Could you check a few things on this model? Use its own coordinates, in mm. Face numbers are marked on the shaded views. A direction names the side the tool comes from. Coordinates: 2 decimals unless noted, no trailing zeros. Loops run counter-clockwise (first coordinate to the right, second up) from the corner with the lowest first, then second, coordinate; pieces in that order, holes last. Notation, with made-up numbers: (56, -16.5) - (79, -16.5) arc R22 cw to (79, -1.5) - close; hole circle Ø2 at (48.25, -29). An arc over 180 degrees is marked (long way). Put each result on its own line as item: value. Start each with the question number.
```python
from build123d import *

# Parameters (mm, degrees)
EXTRUDE_1_DEPTH     = 1.5
EXTRUDE_2_DEPTH     = 3
SKETCH_5_R          = 1.25
CUT_EXTRUDE_2_DEPTH = 2.5000001
CUT_EXTRUDE_3_DEPTH = 2.5000001


with BuildPart() as part:
    # Эскиз1 → Бобышка-Вытянуть1 (new body)
    with BuildSketch(Plane(origin=(0, 0, 0), x_dir=(1, 0, 0), z_dir=(0, 1, 0))):
        with BuildLine():
            Line((5, 14.5), (-5, 14.5))
            ThreePointArc((-5, 14.5), (-9.453000697, 12.420644275), (-13, 9.018919508))
            Line((-13, 9.018919508), (-13, 6.5))
            add(Edge.make_bspline(
                [(-13, 6.5), (-7.441418368, 0), (-13, -6.5)],
                knots=[0, 0, 0, 1, 1, 1], degree=2))
            Line((-13, -6.5), (-13, -9.018919508))
            ThreePointArc((-13, -9.018919508), (-9.453000697, -12.420644275), (-5, -14.5))
            Line((-5, -14.5), (5, -14.5))
            ThreePointArc((5, -14.5), (15.997963501, 0), (5, 14.5))
        make_face()
    extrude(amount=EXTRUDE_1_DEPTH)

    # Эскиз3 → Бобышка-Вытянуть2 (add)
    with BuildSketch(Plane(origin=(0, 1.5, 0), x_dir=(1, 0, 0), z_dir=(0, 1, 0))):
        with BuildLine():
            Line((4.668952027, -11), (7.497379152, -8.171572875))
            Line((7.497379152, -8.171572875), (7.497379152, 8.171572875))
            Line((7.497379152, 8.171572875), (4.668952027, 11))
            Line((4.668952027, 11), (-5.566129175, 11))
            Line((-5.566129175, 11), (-7.502620848, 7.5))
            add(Edge.make_bspline(
                [(-7.502620848, 7.5), (-4.502620848, 0), (-7.502620848, -7.5)],
                knots=[0, 0, 0, 1, 1, 1], degree=2))
            Line((-7.502620848, -7.5), (-5.566129175, -11))
            Line((-5.566129175, -11), (4.668952027, -11))
        make_face()
    extrude(amount=EXTRUDE_2_DEPTH)

    # Эскиз5 → Вырез-Вытянуть2 (cut, through all)
    with BuildSketch(Plane(origin=(0, 1.5, 0), x_dir=(1, 0, 0), z_dir=(0, 1, 0))):
        with Locations((9.863113254, 10.081034519)):
            Circle(SKETCH_5_R)
        with Locations((-10.997789514, 8.218757238)):
            Circle(SKETCH_5_R)
        with Locations((9.863113254, -10.081034519)):
            Circle(SKETCH_5_R)
        with Locations((-10.997789514, -8.218757238)):
            Circle(SKETCH_5_R)
    extrude(amount=-CUT_EXTRUDE_2_DEPTH, mode=Mode.SUBTRACT)

    # Эскиз7 → Вырез-Вытянуть3 (cut, through all)
    with BuildSketch(Plane(origin=(0, 1.5, 0), x_dir=(1, 0, 0), z_dir=(0, 1, 0))):
        with BuildLine():
            Line((-13, 9.018919508), (-13, 6.5))
            Line((-13, 6.5), (-12.715649732, 6.077566297))
            ThreePointArc((-12.715649732, 6.077566297), (-8.737112762, 11.411761045), (-2.842609373, 14.5))
            Line((-2.842609373, 14.5), (-5, 14.5))
            ThreePointArc((-5, 14.5), (-9.453000697, 12.420644275), (-13, 9.018919508))
        make_face()
        with BuildLine():
            Line((-13, -6.5), (-13, -9.018919508))
            ThreePointArc((-13, -9.018919508), (-9.453000697, -12.420644275), (-5, -14.5))
            Line((-5, -14.5), (-2.763931787, -14.5))
            ThreePointArc((-2.763931787, -14.5), (-8.693434445, -11.422725682), (-12.695530111, -6.07372117))
            Line((-12.695530111, -6.07372117), (-13, -6.5))
        make_face()
    extrude(amount=-CUT_EXTRUDE_3_DEPTH, mode=Mode.SUBTRACT)


solid = part.part
```
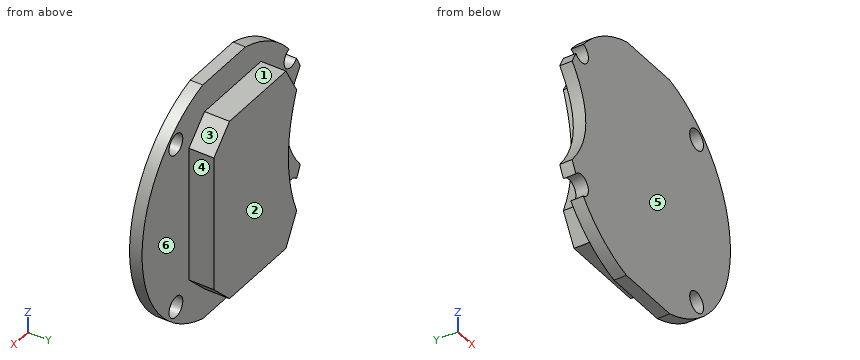
(1) Which directions (+Z, -Z, +X, -X, +Y, -Y) give clear straight access to the entire face, cutting with the end or side of a thin tool? Please do the marked faces 1, 2 and 3.
(2) I want a section at D-D on x = 12. List the corners of the cut face in (y, z) for me, and give its area (3 significant figures).
(3) I want a section at B-B on y = 0.7. Count the separate pieces of the cut face and the enclosed holes in it, and give its area (3 significant figures).
(4) I want a section at A-A on x = 0.25. List the corners of the cut face in (y, z) for me, and give its area (4 significant figures).
(5) I need wall thicknesses on L1, parallel to Y at x = -9.25, z = 9.25; L2, parallel to X at y = 2.35, z = -7.5; L3, parallel to Z at x = -2.5, y = 2.95. Which ranges of each line are inside material? Lowest first, please. Write a range as [from, to].
(6) For pin 1 Ø4 at (x, z) = (9.86, -10.08) entering from -Y; pin 2 Ø1.5 at (x, y) = (6, 1.5) entering from +Z; pin 3 Ø1.5 at (y, z) = (3.5, 2.5) entering from +X; pin 4 Ø1 at (x, y) = (-1, 3) entering from -Z, each with a flat end and sliding along its axis, tell me the tip position at first contact or that it passes through.
(7) I want a section at C-C on x = 6.5. List the corners of the cut face in (y, z) for me.
(8) If we mould it in two halves opening along Y, with no side actions, what happens to the marked faces 4, 5 and 6? For each: pulls with the +Y half, pulls with the -Y half, needs draft (parallel to the pull), parting line crosses it, or undercut.
Answer sheet:
1. face 1: +Z, +X, -X, +Y
1. face 2: +Z, -Z, +X, -X, +Y
1. face 3: +Z, +X, +Y
2. outline: (0, -10.22) - (1.5, -10.22) - (1.5, 10.22) - (0, 10.22) - close
2. area: 30.7 mm^2
3. separate pieces: 1
3. enclosed holes: 2
3. area: 654 mm^2
4. outline: (0, -14.5) - (1.5, -14.5) - (1.5, -11) - (4.5, -11) - (4.5, 11) - (1.5, 11) - (1.5, 14.5) - (0, 14.5) - close
4. area: 109.5 mm^2
5. L1: y = [0, 1.5]
5. L2: x = [-7.5, 7.5]
5. L3: z = [-11, 11]
6. pin 1: stops at y = 0
6. pin 2: stops at z = 14.43
6. pin 3: stops at x = 7.5
6. pin 4: stops at z = -11
7. outline: (0, -13.99) - (1.5, -13.99) - (1.5, -9.17) - (4.5, -9.17) - (4.5, 9.17) - (1.5, 9.17) - (1.5, 13.99) - (0, 13.99) - close
8. face 4: needs draft
8. face 5: pulls with the -Y half
8. face 6: pulls with the +Y half
